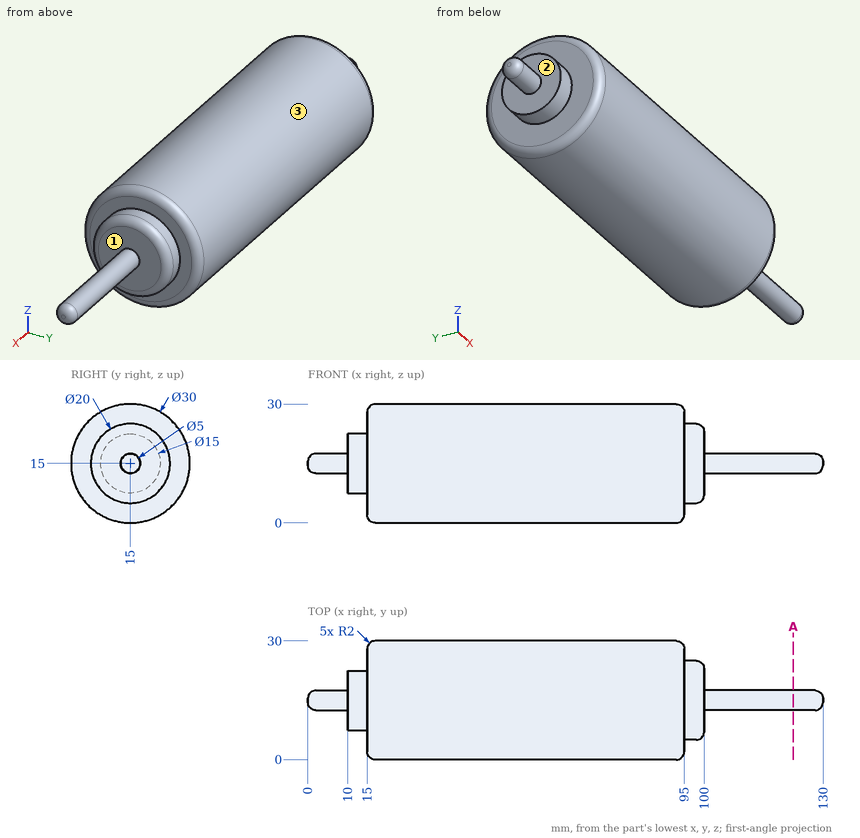
Here's the drawing with two shaded views (mm, measured from the low corner). I have some questions. A direction names the side the tool comes from. Give positions to 0.01 mm unless a question says otherwise; leave off trailing zeros. Order: outer loops, then holes, each group sorted by start corner. A loop starts at its lowest first (then second) coordinate and runs counter-clockwise, first axis right, second up. Notation, with made-up numbers: M 19.5,34.5 L 40.5,34.5 A32 ccw 40.5,68.5 Z; hole C -30,3 d7. An arc over 180 degrees is marked long. One line per item, written item: value.
1) I want a section at A-A, the plane x = 122.5. List the corners of the cut face in (y, z) for me, plus the area to 3 significant figures.
Answer sheet:
outline: C 15,15 d5
area: 19.6 mm^2
2) Please list where these lines run through material, in increasing order: line 1 along X through (y, z) = (24, 8.25); line 2 along X through (y, z) = (21, 19.25); line 3 along Y through (x, z) = (80.5, 15.25).
Answer sheet:
line 1: x = 15 to 95
line 2: x = 10 to 100
line 3: y = 0 to 30
3) On a 3-axis mill with a long thin cutter (end or side, diameter ignored), from which of +Z, -Z, +X, -X, +Y, -Y can I reach the whole of each face in a straight line? I mean the marked faces 1, 2 and 3. Say none if no direction works.
Answer sheet:
face 1: +X
face 2: -X
face 3: +X, -X
4) For P1, Ø8, axis at y = 17, z = 26.5, coming from the +X side; P2, Ø1, axis at x = 33.5, z = 20, coming from the -Y side; P3, Ø5, axis at y = 23, z = 7, coming from the -X side, each with a flat end and sliding along its axis, tell me the tip position at first contact or that it passes through.
Answer sheet:
P1: stops at x = 100
P2: stops at y = 0.69
P3: stops at x = 15
